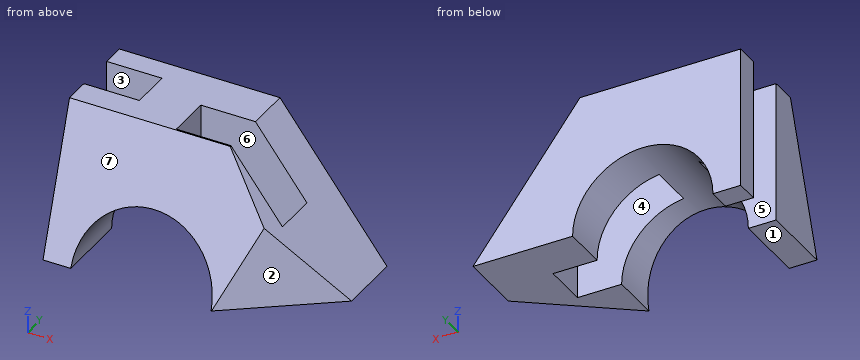
from build123d import *

# Parameters (mm, degrees)
F1_DEPTH       = 84
F3_W           = 33.4407976411
F3_H           = 27
F3_W_2         = 31.5592023589
F4_DEPTH       = 184
F5_W           = 34
F5_H           = 25
F6_DEPTH       = 363
F8_DEPTH       = 191
F13_DEPTH      = 133.5
F13_DEPTH_BACK = 142.2
F15_DEPTH      = 289
F15_DEPTH_BACK = 99


with BuildPart() as f1:
    # F0 (on Front) → F1 (new body)
    with BuildSketch(Plane.XZ):
        Polygon((26.1924322695, 48.2902998924), (-72.2483653716, 48.2902998924), (-72.2483653716, -38.7097001076), (91.7516346284, -38.7097001076), align=None)
    extrude(amount=F1_DEPTH)

    # F3 (on offset) → F4 (cut)
    with BuildSketch(Plane.XY.offset(73.2902998924)):
        with Locations((9.4720334489, -40.5)):
            Rectangle(F3_W, F3_H)
        with Locations((41.9720334489, -40.5)):
            Rectangle(F3_W_2, F3_H)
    extrude(amount=-F4_DEPTH, mode=Mode.SUBTRACT)

    # F5 (on face) → F6 (cut)
    with BuildSketch(Plane.XY.offset(48.2902998924)):
        with Locations((-55.2483653716, -26.5)):
            Rectangle(F5_W, F5_H)
    extrude(amount=-F6_DEPTH, mode=Mode.SUBTRACT)

    # F7 (on face) → F8 (cut)
    with BuildSketch(Plane.XZ.offset(84)):
        with BuildLine():
            ThreePointArc((-55.2483653716, -38.7097001076), (-12.2483653716, -81.7097001076), (30.7516346284, -38.7097001076))
            ThreePointArc((30.7516346284, -38.7097001076), (-12.2483653716, 4.2902998924), (-55.2483653716, -38.7097001076))
        make_face()
    extrude(amount=-F8_DEPTH, mode=Mode.SUBTRACT)

    # F12 (on Right) → F13 (cut, two sides)
    with BuildSketch(Plane.YZ) as f13_sk:
        Polygon((-84, 4.2902998924), (-84, -38.7097001076), (-54.8107397577, 48.2902998924), (-84, 48.2902998924), align=None)
    extrude(amount=-F13_DEPTH, mode=Mode.SUBTRACT)
    extrude(f13_sk.sketch, amount=F13_DEPTH_BACK, mode=Mode.SUBTRACT)

    # F14 (on Top) → F15 (cut, two sides)
    with BuildSketch(Plane.XY) as f15_sk:
        Polygon((91.7516346284, -84), (91.7516346284, -64), (91.7516346284, -39), (30.9858489782, -84), align=None)
    extrude(amount=F15_DEPTH, mode=Mode.SUBTRACT)
    extrude(f15_sk.sketch, amount=-F15_DEPTH_BACK, mode=Mode.SUBTRACT)


solid = f1.part
Design review of the part built by this model. Coordinates are the model's own, in mm. Face numbers are marked on the shaded views. A direction names the side the tool comes from. Give positions to 0.01 mm unless a question says otherwise; leave off trailing zeros. Write each loop counter-clockwise with the first axis right and the second up, starting at its lowest first coordinate (ties: lowest second). Pieces come first, ordered by that corner, then holes. Notation, with made-up numbers: M 40,-6 L 47,-6 A24 ccw 47,17 Z; hole C 18.25,22.25 d6. An arc over 180 degrees is marked long. Answer as a JSON object with one key per item and string values. Group by question number.
1) We need section A-A (y = -42). Give the boundary of the cut face in (x, z), and give its area (3 significant figures).
2) We need section D-D (z = 24.5). Give the boundary of the cut face in (x, y), and give its area (3 significant figures).
3) We need section C-C (y = -19). Give the boundary of the cut face in (x, z).
4) Tool access review of the marked faces 5, 6 and 7: name each direction out of +Z, -Z, +X, -X, +Y, -Y from which nothing blocks a thin tool from reaching the whole face with its end or side.
5) For line 1 along Y through (x, z) = (-53, -22.5); line 2 along X through (y, z) = (-15.5, -3.5); line 3 along X through (y, z) = (-9, -30), list the stretches that pass through material, from the lowest coordinate up.
6) Mouldability with a two-part tool opening along Y and no side actions: class the marked faces 1, 2, 3 and 4 as released by +Y, released by -Y, zero draft, split by the parting line, or undercut.
7) Clearance check with flat-ended pins moving along their axes: pin 1 Ø21.5 at (y, z) = (-40, 16) entering from +X; pin 2 Ø12.5 at (y, z) = (-28.5, 32) entering from -X; pin 3 Ø1 at (y, z) = (-32.5, 17.5) entering from +X; pin 4 Ø1.5 at (y, z) = (-65.5, 25) entering from +X. State where each tip first meets the part, or that it passes through.
8) We need section B-B (z = -14.5). Give the boundary of the cut face in (x, y).
Answer key:
{
 "1": {"outline": "M -72.25,-38.71 L -55.25,-38.71 A43 cw -7.25,4 L -7.25,48.29 L -72.25,48.29 Z; M 57.75,-38.71 L 87.7,-38.71 L 87.7,-33.33 L 57.75,6.41 Z", "area": "4,740 mm²"},
 "2": {"outline": "M -72.25,-62.79 L 44.12,-62.79 L 44.12,-54 L -7.25,-54 L -7.25,-27 L 44.12,-27 L 44.12,0 L -72.25,0 L -72.25,-14 L -38.25,-14 L -38.25,-39 L -72.25,-39 Z", "area": "5,070 mm²"},
 "3": {"outline": "M -38.25,-4.46 A43 cw 30.75,-38.71 L 91.75,-38.71 L 26.19,48.29 L -38.25,48.29 Z"},
 "4": {"face 5": "+Z, -Z, -X", "face 6": "+Z, -Z", "face 7": "+Z, +X, -X, -Y"},
 "5": {"line 1": "y = -78.56 to -39, -14 to 0", "line 2": "x = -38.25 to -36.93, 12.44 to 65.22", "line 3": "x = -72.25 to -54.36, 29.86 to 85.19"},
 "6": {"face 1": "zero draft", "face 2": "released by -Y", "face 3": "undercut", "face 4": "undercut"},
 "7": {"pin 1": "stops at x = 58.63", "pin 2": "stops at x = -38.25", "pin 3": "stops at x = -7.25", "pin 4": "passes through"},
 "8": {"outline": "M -72.25,-75.88 L -47.79,-75.88 L -47.79,-39 L -72.25,-39 Z; M -72.25,-14 L -47.79,-14 L -47.79,0 L -72.25,0 Z; M 23.29,-75.88 L 41.95,-75.88 L 73.51,-52.51 L 73.51,0 L 23.29,0 L 23.29,-27 L 57.75,-27 L 57.75,-54 L 23.29,-54 Z"}
}
